Work out the finished part from the listing and answer in its coordinate system (mm). Face numbers are marked on the shaded views. A direction names the side the tool comes from. Round coordinates to 2 decimals unless told otherwise and drop trailing zeros. Write each loop counter-clockwise with the first axis right and the second up, starting at its lowest first coordinate (ties: lowest second). Pieces come first, ordered by that corner, then holes.
1. Flat-ended cylindrical pins translate along their axes: pin 1 Ø2.5 at (y, z) = (14, 7.5) entering from +X; pin 2 Ø10 at (x, y) = (10, 52.5) entering from -Z; pin 3 Ø2 at (x, z) = (-12, 12.5) entering from +Y. Find the tip coordinate at first contact, or state that the pin passes through.
2. Find section D-D (y = 55.5). Write down the section's boundary in (x, z).
3. Determine the mould class of the marked faces 1, 2, 3 and 4 for opening direction Y: pulls with the +Y half, pulls with the -Y half, needs draft (parallel to the pull), parting line crosses it, or undercut.
4. A tool of negligible diameter and unlimited length cuts with its end or side. For the marked faces 5, 6 and 7, from which of +Z, -Z, +X, -X, +Y, -Y can it reach the whole face along a straight path? Write none if from no direction.
5. Find section C-C (x = 12). Write down the section's boundary in (y, z).
6. Find section A-A (z = 3.25). Count the separate pieces of the cut face and the enclosed holes in it, and give its area (3 significant figures).
7. Straight lines are drawn through the part: probe 1 along Y at (x, z) = (0, 2.25); probe 2 along Y at (x, z) = (7, 7); probe 3 along Z at (x, y) = (-9, 50). For each, find the intervals that lie inside material, in ascending order.
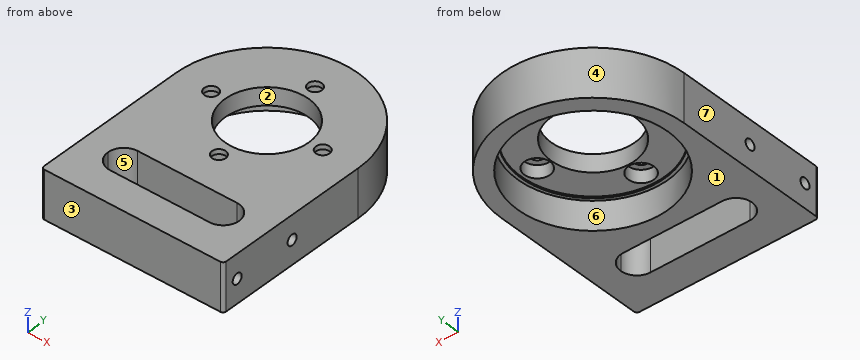
```python
from build123d import *

# Parameters (mm, degrees)
SKETCH_1_R           = 13.1
SKETCH_1_R_2         = 2.15
EXTRUDE_1_DEPTH      = 15
SKETCH_2_R           = 1.65
CUT_EXTRUDE_2_DEPTH  = 10
FILLET_3_R           = 1
SKETCH_7_R           = 23.5
CUT_EXTRUDE_7_DEPTH  = 9
SKETCH_9_R           = 22.5
CUT_EXTRUDE_9_DEPTH  = 0.5
SKETCH_10_R          = 4
CUT_EXTRUDE_10_DEPTH = 4
CUT_EXTRUDE_11_DEPTH = 80.771072474
SKETCH_12_W          = 41.12
SKETCH_12_H          = 10
CUT_EXTRUDE_12_DEPTH = 74.965581185
FILLET_4_R           = 5


with BuildPart() as part:
    # ｽｹｯﾁ1 → ﾎﾞｽ - 押し出し1 (new body)
    with BuildSketch(Plane.XY):
        with BuildLine():
            Line((-28.56, -11), (28.56, -11))
            Line((28.56, -11), (28.56, 21.386752274))
            ThreePointArc((28.56, 21.386752274), (0, 71.040484258), (-28.56, 21.386752274))
            Line((-28.56, 21.386752274), (-28.56, -11))
        make_face()
        with Locations((0, 38)):
            Circle(SKETCH_1_R, mode=Mode.SUBTRACT)
        with Locations((0, 55.5)):
            Circle(SKETCH_1_R_2, mode=Mode.SUBTRACT)
        with Locations((17.5, 38)):
            Circle(SKETCH_1_R_2, mode=Mode.SUBTRACT)
        with Locations((0, 20.5)):
            Circle(SKETCH_1_R_2, mode=Mode.SUBTRACT)
        with Locations((-17.5, 38)):
            Circle(SKETCH_1_R_2, mode=Mode.SUBTRACT)
    extrude(amount=EXTRUDE_1_DEPTH)

    # ｽｹｯﾁ2 → ｶｯﾄ - 押し出し2 (cut)
    with BuildSketch(Plane(origin=(28.56, 0, 0), x_dir=(0, 0, -1), z_dir=(1, 0, 0))):
        with Locations((-7.5, -6)):
            Circle(SKETCH_2_R)
        with Locations((-7.5, 14)):
            Circle(SKETCH_2_R)
    cut_extrude_2 = extrude(amount=-CUT_EXTRUDE_2_DEPTH, mode=Mode.SUBTRACT)

    # ﾐﾗｰ2: ｶｯﾄ - 押し出し2 across plane
    add(cut_extrude_2.mirror(Plane.ZY), mode=Mode.SUBTRACT)

    # ﾌｨﾚｯﾄ3
    fillet_3_edges = [part.edges().sort_by_distance(p)[0] for p in [
        (28.56, -11, 7.5),
        (-28.56, -11, 7.5),
    ]]
    fillet(fillet_3_edges, radius=FILLET_3_R)

    # ｽｹｯﾁ7 → ｶｯﾄ - 押し出し7 (cut)
    with BuildSketch(Plane(origin=(0, 0, 0), x_dir=(-1, 0, 0), z_dir=(0, 0, -1))):
        with Locations((0, 38)):
            Circle(SKETCH_7_R)
    extrude(amount=-CUT_EXTRUDE_7_DEPTH, mode=Mode.SUBTRACT)

    # ｽｹｯﾁ9 → ｶｯﾄ - 押し出し9 (cut)
    with BuildSketch(Plane(origin=(0, 0, 9), x_dir=(-1, 0, 0), z_dir=(0, 0, -1))):
        with Locations((0, 38)):
            Circle(SKETCH_9_R)
    extrude(amount=-CUT_EXTRUDE_9_DEPTH, mode=Mode.SUBTRACT)

    # ｽｹｯﾁ10 → ｶｯﾄ - 押し出し10 (cut)
    with BuildSketch(Plane(origin=(0, 0, 9.5), x_dir=(-1, 0, 0), z_dir=(0, 0, -1))):
        with Locations((0, 55.5)):
            Circle(SKETCH_10_R)
        with Locations((17.5, 38)):
            Circle(SKETCH_10_R)
        with Locations((-17.5, 38)):
            Circle(SKETCH_10_R)
        with Locations((0, 20.5)):
            Circle(SKETCH_10_R)
    extrude(amount=-CUT_EXTRUDE_10_DEPTH, mode=Mode.SUBTRACT)

    # ｽｹｯﾁ11 → ｶｯﾄ - 押し出し11 (cut, through all)
    with BuildSketch(Plane(origin=(0, 0, 0), x_dir=(-1, 0, 0), z_dir=(0, 0, -1))):
        with BuildLine():
            Line((-28.56, 21.386752274), (-28.56, 38))
            ThreePointArc((-28.56, 38), (0, 66.56), (28.56, 38))
            Line((28.56, 38), (28.56, 21.386752274))
            ThreePointArc((28.56, 21.386752274), (31.900703992, 29.39658877), (33.040484258, 38))
            ThreePointArc((33.040484258, 38), (-8.60341123, 69.900703992), (-28.56, 21.386752274))
        make_face()
    extrude(amount=-CUT_EXTRUDE_11_DEPTH, mode=Mode.SUBTRACT)

    # ｽｹｯﾁ12 → ｶｯﾄ - 押し出し12 (cut, through all)
    with BuildSketch(Plane(origin=(0, 0, 0), x_dir=(-1, 0, 0), z_dir=(0, 0, -1))):
        with Locations((0, 4)):
            Rectangle(SKETCH_12_W, SKETCH_12_H)
    extrude(amount=-CUT_EXTRUDE_12_DEPTH, mode=Mode.SUBTRACT)

    # ﾌｨﾚｯﾄ4
    fillet_4_edges = [part.edges().sort_by_distance(p)[0] for p in [
        (-20.56, 9, 7.5),
        (-20.56, -1, 7.5),
        (20.56, 9, 7.5),
        (20.56, -1, 7.5),
    ]]
    fillet(fillet_4_edges, radius=FILLET_4_R - 0.0001)  # a hair under: the kernel refuses the full size


solid = part.part
```
Worked answers:
1. pin 1: stops at x = 18.56
1. pin 2: stops at z = 9
1. pin 3: stops at y = 64.36
2. outline: (-22.57, 0) - (-15.68, 0) - (-15.68, 9) - (-14.14, 9) - (-14.14, 9.5) - (-4, 9.5) - (-4, 13.5) - (-2.15, 13.5) - (-2.15, 15) - (-22.57, 15) - close; (2.15, 13.5) - (4, 13.5) - (4, 9.5) - (14.14, 9.5) - (14.14, 9) - (15.68, 9) - (15.68, 0) - (22.57, 0) - (22.57, 15) - (2.15, 15) - close
3. face 1: needs draft
3. face 2: undercut
3. face 3: pulls with the -Y half
3. face 4: pulls with the +Y half
4. face 5: +Z, -Z
4. face 6: -Z
4. face 7: +Z, -Z, -X, +Y, -Y
5. outline: (-11, 0) - (-1, 0) - (-1, 15) - (-11, 15) - close; (9, 0) - (17.79, 0) - (17.79, 9) - (18.97, 9) - (18.97, 9.5) - (32.75, 9.5) - (32.75, 15) - (9, 15) - close; (43.25, 9.5) - (57.03, 9.5) - (57.03, 9) - (58.21, 9) - (58.21, 0) - (63.92, 0) - (63.92, 15) - (43.25, 15) - close
6. separate pieces: 1
6. enclosed holes: 2
6. area: 1,960 mm2
7. probe 1: y = -11 to -1, 9 to 14.5, 61.5 to 66.56
7. probe 2: y = -11 to -1, 9 to 15.57, 60.43 to 65.69
7. probe 3: z = 9.5 to 15
